```python
from build123d import *

# Parameters (mm, degrees)
SALIENTE_EXTRUIR1_DEPTH       = 95.25
TALADRO_DE_MARGEN_PARA_1_41_D = 6.7564


with BuildPart() as part:
    # Croquis1 → Saliente-Extruir1 (new, symmetric)
    with BuildSketch(Plane.XY):
        Polygon((-1.35, -25), (6.35, -5), (6.35, 25), (-6.35, 25), (-6.35, -25), align=None)
    extrude(amount=SALIENTE_EXTRUIR1_DEPTH, both=True)

    # Taladro de margen para 1/41 (through all)
    with Locations(Plane(origin=(6.35, 0, 0), x_dir=(0, 0, -1), z_dir=(1, 0, 0))):
        with Locations((-45.25, 0), (45.25, 0)):
            Hole(TALADRO_DE_MARGEN_PARA_1_41_D / 2)

    # Croquis7 → Taladro roscado 3/8-161 (revolve, cut)
    with BuildSketch(Plane(origin=(6.35, 15, 0), x_dir=(0, 0, -1), z_dir=(0, 1, 0))):
        Polygon((0, 0), (0, 12.7), (5.3975, 12.7), (3.96875, 11.27125), (3.96875, 1.42875), (5.3975, 0), align=None)
    revolve(axis=Axis((12.7, 15, 0), (-1, 0, 0)), mode=Mode.SUBTRACT)


solid = part.part
```
Check sheet for the modelled part. Datum: model origin and axes. Units: mm. Round coordinates to 2 decimals unless told otherwise and drop trailing zeros. Loops run counter-clockwise (first coordinate to the right, second up) from the corner with the lowest first, then second, coordinate; pieces in that order, holes last. Notation, with made-up numbers: (72, 31.5) -> (128, 31.5) arc R10 cw to (128, 42.5) -> close; hole circle Ø1 at (-39.5, 71). An arc over 180 degrees is marked (long way). Answer in a Markdown table with one row per item.
Q1. Thickness scan on L1, parallel to Z at x = 0, y = 15; L2, parallel to Y at x = -2.5, z = -45.25; L3, parallel to Z at x = 2, y = -1. Record the ranges inside material, lowest first.
Data:
| item | result |
|---|---|
| L1 | z = -95.25 to -3.97, 3.97 to 95.25 |
| L2 | y = -25 to -3.38, 3.38 to 25 |
| L3 | z = -95.25 to -48.48, -42.02 to 42.02, 48.48 to 95.25 |
Q2. Sectioned sample at D-D on x = 1.5. Enter the section's corners in (y, z).
Data:
| item | result |
|---|---|
| outline | (-17.6, -95.25) -> (25, -95.25) -> (25, 95.25) -> (-17.6, 95.25) -> close; hole circle Ø6.76 at (0, -45.25); hole circle Ø6.76 at (0, 45.25); hole circle Ø7.94 at (15, 0) |
Q3. Sectioned sample at B-B on y = 0. Enter the section's corners in (x, z).
Data:
| item | result |
|---|---|
| outline | (-6.35, -95.25) -> (6.35, -95.25) -> (6.35, -48.63) -> (-6.35, -48.63) -> close; (-6.35, -41.87) -> (6.35, -41.87) -> (6.35, 41.87) -> (-6.35, 41.87) -> close; (-6.35, 48.63) -> (6.35, 48.63) -> (6.35, 95.25) -> (-6.35, 95.25) -> close |
Q4. Go/stop test with a flat-tipped pin: P1, Ø10.5, axis at y = 15, z = 0, coming from the -X side. Record where the tip stops, or that it passes through.
Data:
| item | result |
|---|---|
| P1 | stops at x = -6.2 |
Q5. Sectioned sample at A-A on z = 0. Enter the section's corners in (x, y), then the cut area to 3 significant figures.
Data:
| item | result |
|---|---|
| outline | (-6.35, -25) -> (-1.35, -25) -> (6.35, -5) -> (6.35, 9.6) -> (4.92, 11.03) -> (-4.92, 11.03) -> (-6.35, 9.6) -> close; (-6.35, 20.4) -> (-4.92, 18.97) -> (4.92, 18.97) -> (6.35, 20.4) -> (6.35, 25) -> (-6.35, 25) -> close |
| area | 453 mm^2 |
Q6. Sectioned sample at C-C on z = -45.25. Enter the section's corners in (x, y).
Data:
| item | result |
|---|---|
| outline | (-6.35, -25) -> (-1.35, -25) -> (6.35, -5) -> (6.35, -3.38) -> (-6.35, -3.38) -> close; (-6.35, 3.38) -> (6.35, 3.38) -> (6.35, 25) -> (-6.35, 25) -> close |
Q7. Release check for a two-part mould opening along Y. For faces 1 (the face through (0, 0, -95.25)), 2 (the face through (0, 25, 1)), 3 (the face through (0.069, 11.065, 0.517)) record: released by +Y, released by -Y, zero draft, split by the parting line, or undercut.
Data:
| item | result |
|---|---|
| face 1 | zero draft |
| face 2 | released by +Y |
| face 3 | undercut |
